```python
from build123d import *

# Parameters (mm, degrees)
F0_R     = 9.95
F0_R_2   = 11
F1_DEPTH = 3


with BuildPart() as f1:
    # F0 (on Top) → F1 (new body)
    with BuildSketch(Plane.XY):
        with BuildLine():
            ThreePointArc((-3, -20.234534), (-0.51911, -49.97929), (3, -20.339432))
            Line((3, -20.339432), (3, -14.661455))
            ThreePointArc((3, -14.661455), (10.582019, -10.582019), (14.661455, -3))
            Line((14.661455, -3), (20.302832, -3))
            ThreePointArc((20.302832, -3), (50, -0.002273), (20.303291, 3))
            Line((20.303291, 3), (14.661455, 3))
            ThreePointArc((14.661455, 3), (10.582019, 10.582019), (3, 14.661455))
            Line((3, 14.661455), (3, 20.339432))
            ThreePointArc((3, 20.339432), (-0.51911, 49.97929), (-3, 20.234534))
            Line((-3, 20.234534), (-3, 14.661455))
            ThreePointArc((-3, 14.661455), (-10.582019, 10.582019), (-14.661455, 3))
            Line((-14.661455, 3), (-20.303291, 3))
            ThreePointArc((-20.303291, 3), (-50, -0.002273), (-20.302832, -3))
            Line((-20.302832, -3), (-14.661455, -3))
            ThreePointArc((-14.661455, -3), (-10.582019, -10.582019), (-3, -14.661455))
            Line((-3, -14.661455), (-3, -20.234534))
        make_face()
        with Locations((-35, -0.001125)):
            Circle(F0_R, mode=Mode.SUBTRACT)
        with Locations((0, -35)):
            Circle(F0_R, mode=Mode.SUBTRACT)
        with Locations((35, -0.001125)):
            Circle(F0_R, mode=Mode.SUBTRACT)
        Circle(F0_R_2, mode=Mode.SUBTRACT)
        with Locations((0, 35)):
            Circle(F0_R, mode=Mode.SUBTRACT)
    extrude(amount=F1_DEPTH)


solid = f1.part
```
CAD build for the part. Positions are in the model's coordinates, mm. Round coordinates to 2 decimals unless told otherwise and drop trailing zeros. Write each loop counter-clockwise with the first axis right and the second up, starting at its lowest first coordinate (ties: lowest second). Pieces come first, ordered by that corner, then holes. Notation, with made-up numbers: (-23, -24.5) - (30, -24.5) arc R17 ccw to (30, -18.5) - close; hole circle Ø7 at (-1.5, 54). An arc over 180 degrees is marked (long way). Return JSON: item names as keys, results as strings. Group by question number.
Item 1: Band-saw the part on A-A on x = -35. List the corners of the cut face in (y, z), plus the area to 3 significant figures.
Item 2: Probe probe 1 along Y at (x, z) = (0, 0.7); probe 2 along X at (y, z) = (12.5, 1.55); probe 3 along X at (y, z) = (-13, 1.9). List the from-to ranges inside material, lowest first.
Item 3: Mould opens along X. For faces 1 (the face through (-1.136, -49.956, 1.479)), 2 (the face through (-8, -11, 3)), 3 (the face through (-17, 3, 1)) say: +X half, -X half, draft (parallel to the pull), parting line (faces both ways), or undercut.
Item 4: Band-saw the part on B-B on y = -1.5. List the corners of the cut face in (x, z).
Item 5: Flat gauge pins, fed straight in: pin 1 Ø1 at (x, z) = (-18.5, 1.5) entering from +Y; pin 2 Ø0.9 at (y, z) = (-17, 2) entering from -X; pin 3 Ø3 at (x, y) = (-8, 31) entering from -Z; pin 4 Ø17.5 at (x, y) = (0, 0) entering from +Z. Where does each tip first touch, or does it go through?
Item 6: Band-saw the part on D-D on z = 1.25. List the corners of the cut face in (x, y).
Item 7: Band-saw the part on C-C on x = 0. List the corners of the cut face in (y, z).
Resolved:
{
 "1": {"outline": "(-15, 0) - (-9.95, 0) - (-9.95, 3) - (-15, 3) - close; (9.95, 0) - (15, 0) - (15, 3) - (9.95, 3) - close", "area": "30.3 mm²"},
 "2": {"probe 1": "y = -49.98 to -44.95, -25.05 to -11, 11 to 25.05, 44.95 to 49.98", "probe 2": "x = -43.29 to -26.71, -8.23 to 8.23, 26.71 to 43.29", "probe 3": "x = -42.49 to -27.51, -7.41 to 7.41, 27.51 to 42.49"},
 "3": {"face 1": "parting line", "face 2": "draft", "face 3": "undercut"},
 "4": {"outline": "(-49.92, 0) - (-44.84, 0) - (-44.84, 3) - (-49.92, 3) - close; (-25.16, 0) - (-10.9, 0) - (-10.9, 3) - (-25.16, 3) - close; (10.9, 0) - (25.16, 0) - (25.16, 3) - (10.9, 3) - close; (44.84, 0) - (49.92, 0) - (49.92, 3) - (44.84, 3) - close"},
 "5": {"pin 1": "stops at y = 3", "pin 2": "stops at x = -3", "pin 3": "stops at z = 0", "pin 4": "passes through"},
 "6": {"outline": "(-20.3, -3) - (-14.66, -3) arc R14.97 ccw to (-3, -14.66) - (-3, -20.23) arc R15 ccw (long way) to (3, -20.34) - (3, -14.66) arc R14.97 ccw to (14.66, -3) - (20.3, -3) arc R15 ccw (long way) to (20.3, 3) - (14.66, 3) arc R14.97 ccw to (3, 14.66) - (3, 20.34) arc R15 ccw (long way) to (-3, 20.23) - (-3, 14.66) arc R14.97 ccw to (-14.66, 3) - (-20.3, 3) arc R15 ccw (long way) to start; hole circle Ø19.9 at (-35, 0); hole circle Ø22 at (0, 0); hole circle Ø19.9 at (0, -35); hole circle Ø19.9 at (0, 35); hole circle Ø19.9 at (35, 0)"},
 "7": {"outline": "(-49.98, 0) - (-44.95, 0) - (-44.95, 3) - (-49.98, 3) - close; (-25.05, 0) - (-11, 0) - (-11, 3) - (-25.05, 3) - close; (11, 0) - (25.05, 0) - (25.05, 3) - (11, 3) - close; (44.95, 0) - (49.98, 0) - (49.98, 3) - (44.95, 3) - close"}
}
